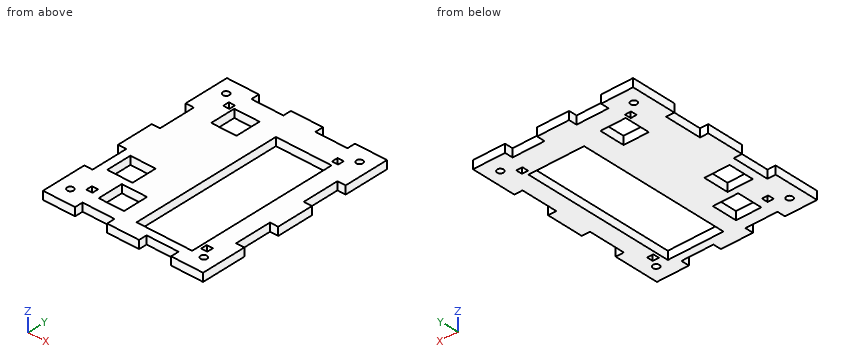
Autodesk Inventor part; units mm, degrees
ref_plane "YZ Plane" through (0, 0, 0) normal (1, 0, 0) x (0, 1, 0)
ref_plane "XZ Plane" through (0, 0, 0) normal (0, 1, 0) x (-1, 0, 0)
ref_plane "XY Plane" through (0, 0, 0) normal (0, 0, 1) x (1, 0, 0)
sketch "Sketch1" plane through (0, 0, 0) normal (0, 0, 1) x (1, 0, 0)
  line L0 (-39, 49) -> (39, 49)
  line L1 (39, 49) -> (39, -49)
  line L2 (39, -49) -> (-39, -49)
  line L3 (-39, -49) -> (-39, 49)
  line L4 (-23.4, -45) -> (-7.8, -45)
  line L5 (-7.8, -45) -> (-7.8, -49)
  line L6 (-7.8, -49) -> (-23.4, -49)
  line L7 (-23.4, -49) -> (-23.4, -45)
  line L8 (-39, -27) -> (-35, -27)
  line L9 (-35, -27) -> (-35, -9)
  line L10 (-35, -9) -> (-39, -9)
  line L11 (-39, -9) -> (-39, -27)
  line L12 (0, 0) -> (8.9596, 0)
  line L13 (0, 0) -> (0, 8.0367)
  line L14 (-23.4, 45) -> (-7.8, 45)
  line L15 (-7.8, 45) -> (-7.8, 49)
  line L16 (-23.4, 49) -> (-23.4, 45)
  line L17 (-39, 27) -> (-35, 27)
  line L18 (-35, 27) -> (-35, 9)
  line L19 (-35, 9) -> (-39, 9)
  line L20 (23.4, -45) -> (7.8, -45)
  line L21 (7.8, -45) -> (7.8, -49)
  line L22 (23.4, -49) -> (23.4, -45)
  line L23 (39, -27) -> (35, -27)
  line L24 (35, -27) -> (35, -9)
  line L25 (35, -9) -> (39, -9)
  line L26 (0, 0) -> (-8.9596, 0)
  line L27 (39, 27) -> (35, 27)
  line L28 (35, 27) -> (35, 9)
  line L29 (35, 9) -> (39, 9)
  line L30 (7.8, 45) -> (7.8, 49)
  line L31 (23.4, 49) -> (23.4, 45)
  line L32 (23.4, 45) -> (7.8, 45)
  point P0 (0, 49)
  point P1 (39, 0)
  point P2 (0, -49)
  point P3 (-7.8, -47)
  point P4 (-37, -9)
  dimension "d0" = 98
  dimension "d1" = 78
  dimension "d2" = 15.6
  dimension "d3" = 4
  dimension "d4" = 4
  dimension "d5" = 18
  dimension "d6" = 7.8
  dimension "d7" = 9
extrude "Extrusion1" add sketch "Sketch1" along normal mid plane 4 contours L0 L16 L14 L15 L30 L32 L31 L1 L27 L28 L29 L25 L24 L23 L2 L22 L20 L21 L5 L4 L7 L3 L8 L9 L10 L19 L18 L17
sketch "Sketch2" plane through (0, 0, 2) normal (0, 0, 1) x (1, 0, 0)
  line L0 (-21, -39) -> (-8.7, -39)
  line L1 (-8.7, -39) -> (-8.7, -26.7)
  line L2 (-8.7, -26.7) -> (-21, -26.7)
  line L3 (-21, -26.7) -> (-21, -39)
  line L4 (-35, -9) -> (-35, -27)
  line L5 (-23.4, -45) -> (-7.8, -45)
  line L6 (-18.7, -11.2) -> (-31, -11.2)
  line L7 (-31, -11.2) -> (-31, -23.5)
  line L8 (-31, -23.5) -> (-18.7, -23.5)
  line L9 (-18.7, -23.5) -> (-18.7, -11.2)
  line L10 (-11.45, 36.25) -> (-23.75, 36.25)
  line L11 (-23.75, 36.25) -> (-23.75, 23.95)
  line L12 (-23.75, 23.95) -> (-11.45, 23.95)
  line L13 (-11.45, 23.95) -> (-11.45, 36.25)
  line L14 (-7.8, 45) -> (-23.4, 45)
  line L15 (-35, 27) -> (-35, 9)
  line L16 (26.6, 33) -> (-0.5, 33)
  line L17 (-0.5, 33) -> (-0.5, -41.25)
  line L18 (-0.5, -41.25) -> (26.6, -41.25)
  line L19 (26.6, -41.25) -> (26.6, 33)
  line L20 (23.4, 45) -> (7.8, 45)
  circle A0 centre (-32.5, -41.5) radius 1.55
  line L21 (35, 9) -> (35, 27)
  line L22 (0, 0) -> (5.8135, 0)
  line L23 (0, 0) -> (0, 4.2513)
  line L24 (7.8, -45) -> (23.4, -45)
  line L25 (35, -27) -> (35, -9)
  line L26 (-28, -35) -> (-25, -35)
  line L27 (-25, -35) -> (-25, -38)
  line L28 (-25, -38) -> (-28, -38)
  line L29 (-28, -38) -> (-28, -35)
  line L30 (-39, -49) -> (-23.4, -49)
  line L31 (-39, -27) -> (-39, -49)
  circle A1 centre (-32.5, 41.5) radius 1.55
  line L32 (-28, 35) -> (-25, 35)
  line L33 (-25, 35) -> (-25, 38)
  line L34 (-25, 38) -> (-28, 38)
  line L35 (-28, 38) -> (-28, 35)
  line L36 (28, 35) -> (25, 35)
  line L37 (25, 35) -> (25, 38)
  line L38 (28, 38) -> (28, 35)
  line L39 (25, 38) -> (28, 38)
  circle A2 centre (32.5, 41.5) radius 1.55
  circle A3 centre (32.5, -41.5) radius 1.55
  line L40 (28, -35) -> (31, -35)
  line L41 (31, -35) -> (31, -38)
  line L42 (31, -38) -> (28, -38)
  line L43 (28, -38) -> (28, -35)
  line L44 (23.4, -49) -> (39, -49)
  line L45 (39, -49) -> (39, -27)
  point P0 (-17.6, 36.25)
  point P1 (-8.7, -32.85)
  point P2 (-39, -38)
  point P3 (29.5, -38)
  dimension "d10" = 12.3
  dimension "d11" = 12.3
  dimension "d12" = 14
  dimension "d13" = 6
  dimension "d14" = 4
  dimension "d15" = 21.5
  dimension "d16" = 12.3
  dimension "d17" = 12.3
  dimension "d18" = 8.75
  dimension "d19" = 11.25
  dimension "d20" = 12.3
  dimension "d21" = 12.3
  dimension "d24" = 27.1
  dimension "d25" = 34.5
  dimension "d26" = 12
  dimension "d29" = 3.1
  dimension "d30" = 3.5
  dimension "d31" = 2.5
  dimension "d49" = 3
  dimension "d50" = 3
  dimension "d51" = 11
  dimension "d52" = 11
  dimension "d53" = 3
  dimension "d54" = 3
  dimension "d55" = 11
  dimension "d56" = 8
extrude "Extrusion2" cut sketch "Sketch2" against normal up to surface (4 mm away)
equation "\"d11\" = d10"
equation "\"d16\" = d10"
equation "\"d17\" = d10"
equation "\"d20\" = d16"
equation "\"d21\" = d20"
equation "\"d50\" = d49"
properties part number "Top"
Input: part model. Units: mm. Frame: model coordinates. Round coordinates to 2 decimals unless told otherwise and drop trailing zeros. Order: outer loops, then holes, each group sorted by start corner. A loop starts at its lowest first (then second) coordinate and runs counter-clockwise, first axis right, second up. Notation, with made-up numbers: (-33, 51) - (-24, 51) arc R21 cw to (-24, 66) - close; hole circle Ø2 at (17, 55.25). An arc over 180 degrees is marked (long way). Answer in a Markdown table with one row per item.
Item 1: Section query A-A (x = -32.5). Return the cut outline in (y, z), then the cut area to 3 significant figures.
Model answer:
| item | result |
|---|---|
| outline | (-49, -2) - (-43.05, -2) - (-43.05, 2) - (-49, 2) - close; (-39.95, -2) - (39.95, -2) - (39.95, 2) - (-39.95, 2) - close; (43.05, -2) - (49, -2) - (49, 2) - (43.05, 2) - close |
| area | 367 mm² |
Item 2: Line query: line 1 (Y direction, x = -32.5, z = -0.75); line 2 (X direction, y = -12.5, z = 0.35); line 3 (Y direction, x = -22.5, z = -0.4). Output: solid intervals per line, ascending.
Model answer:
| item | result |
|---|---|
| line 1 | y = -49 to -43.05, -39.95 to 39.95, 43.05 to 49 |
| line 2 | x = -35 to -31, -18.7 to -0.5, 26.6 to 35 |
| line 3 | y = -45 to -23.5, -11.2 to 23.95, 36.25 to 45 |
Item 3: Section query B-B (y = -1). Return the cut outline in (x, z).
Model answer:
| item | result |
|---|---|
| outline | (-39, -2) - (-0.5, -2) - (-0.5, 2) - (-39, 2) - close; (26.6, -2) - (39, -2) - (39, 2) - (26.6, 2) - close |
Item 4: Section query D-D (x = 16.5). Return the cut outline in (y, z).
Model answer:
| item | result |
|---|---|
| outline | (-45, -2) - (-41.25, -2) - (-41.25, 2) - (-45, 2) - close; (33, -2) - (45, -2) - (45, 2) - (33, 2) - close |
Item 5: Pin query (flat end, axial travel): pin 1 (2 mm diameter, centred on y = 11.5, z = -0.5, fed in from +X); pin 2 (2 mm diameter, centred on x = 12, z = -1, fed in from -Y). Return the tip coordinate at first contact, or that it passes through.
Model answer:
| item | result |
|---|---|
| pin 1 | stops at x = 35 |
| pin 2 | stops at y = -45 |
Item 6: Section query C-C (y = 41.5). Return the cut outline in (x, z), then the cut area to 3 significant figures.
Model answer:
| item | result |
|---|---|
| outline | (-39, -2) - (-34.05, -2) - (-34.05, 2) - (-39, 2) - close; (-30.95, -2) - (30.95, -2) - (30.95, 2) - (-30.95, 2) - close; (34.05, -2) - (39, -2) - (39, 2) - (34.05, 2) - close |
| area | 287 mm² |
